CAD build for the part. Positions are in the model's coordinates, mm. A direction names the side the tool comes from. Give positions to 0.01 mm unless a question says otherwise; leave off trailing zeros. Order: outer loops, then holes, each group sorted by start corner. A loop starts at its lowest first (then second) coordinate and runs counter-clockwise, first axis right, second up.
Item 1: Band-saw the part on A-A on x = 48. Give the cut face in (y, z), plus the area to 3 significant figures.
Item 2: Band-saw the part on D-D on y = -14. Give the cut face in (x, z).
Item 3: Two-plate mould, pull along X, no slides. Class faces 6 (the flat face through (-3, 0, 6)), 7 (the cylindrical face through (-101.154, -39.08, -32.591)), 8 (the flat face through (-100.039, -47.546, 19.409)): released by +X, released by -X, zero draft, split by the parting line, or undercut.
Item 4: Band-saw the part on C-C on z = 3. Give the cut face in (x, y).
Item 5: Flat gauge pins, fed straight in: P1, Ø12, axis at y = -21, z = -22, coming from the +X side; P2, Ø10.5, axis at x = 25.5, z = 9.5, coming from the -Y side; P3, Ø8, axis at x = 1.5, y = -27.5, coming from the -Z side; P4, Ø5, axis at x = 21.5, y = -37, coming from the -Z side. Where does each tip first touch, or does it go through?
Item 6: Wall check: L1, parallel to Z at x = -92, y = -44; L2, parallel to Z at x = -74.5, y = -15; L3, parallel to Y at x = -19, z = 6. Give the ranges that are in metal, low to high.
Item 7: Which spindle directions (+Z, -Z, +X, -X, +Y, -Y) get a long thin tool onto all of the face, cutting with end or side? Do faces 1 (the flat face through (-95, -39, 15)), 2 (the flat face through (-78.604, -9.86, 19.409)), 3 (the flat face through (-93, -30, 13)), 4 (the flat face through (-78.604, -9.86, -19.227)), 5 (the flat face through (25, -22, 6)). Say none if no direction does.
Item 8: Band-saw the part on B-B on y = -47. Give the cut face in (x, z).
```python
from build123d import *

# Parameters (mm, degrees)
PAD_DEPTH    = 13
PAD001_DEPTH = 13
PAD002_DEPTH = 26
PAD003_DEPTH = 13
SKETCH004_R  = 6
POCKET_DEPTH = 54


with BuildPart() as part:
    # Sketch → Pad (new body)
    with BuildSketch(Plane.XY):
        Polygon((-84.297005, 0), (80.002995, 0), (80.002995, -20), (0, -20), (0, -22), (50, -22), (50, -33), (0, -33), (0, -35), (-5, -35), (-5, -20), (-72.75, -20), (-77.75, -28.660254), (-89.297005, -8.660254), align=None)
    extrude(amount=PAD_DEPTH)

    # Sketch001 (on Face16 of Pad) → Pad001 (join)
    with BuildSketch(Plane.XY.offset(13)):
        Polygon((-84.297005, 0), (-72.75, -20), (-91.5, -52.475953), (-108.820508, -42.475953), align=None)
    extrude(amount=PAD001_DEPTH)

    # Sketch002 (on Face4 of Pad001) → Pad002 (join)
    with BuildSketch(Plane(origin=(0, 0, 0), x_dir=(1, 0, 0), z_dir=(0, 0, -1))):
        Polygon((-77.75, 28.660254), (-89.297005, 8.660254), (-84.297005, 0), (-72.75, 20), align=None)
    extrude(amount=PAD002_DEPTH)

    # Sketch003 (on Face23 of Pad002) → Pad003 (join)
    with BuildSketch(Plane(origin=(0, 0, -26), x_dir=(1, 0, 0), z_dir=(0, 0, -1))):
        Polygon((-72.75, 20), (-91.5, 52.475953), (-108.820508, 42.475953), (-84.297005, 0), align=None)
    extrude(amount=PAD003_DEPTH)

    # Sketch004 (on Face31 of Pad003) → Pocket (cut)
    with BuildSketch(Plane(origin=(0, 0, -39), x_dir=(1, 0, 0), z_dir=(0, 0, -1))):
        with Locations((-95.160254, 38.815699)):
            Circle(SKETCH004_R)
    extrude(amount=-POCKET_DEPTH, mode=Mode.SUBTRACT)


solid = part.part
```
The answers:
1. outline: (-33, 0) - (-22, 0) - (-22, 13) - (-33, 13) - close; (-20, 0) - (0, 0) - (0, 13) - (-20, 13) - close
1. area: 403 mm2
2. outline: (-92.38, -39) - (-76.21, -39) - (-76.21, 0) - (80, 0) - (80, 13) - (-76.21, 13) - (-76.21, 26) - (-92.38, 26) - (-92.38, 13) - (-86.21, 13) - (-86.21, -26) - (-92.38, -26) - close
3. face 6: zero draft
3. face 7: undercut
3. face 8: released by -X
4. outline: (-89.3, -8.66) - (-77.75, -28.66) - (-72.75, -20) - (-5, -20) - (-5, -35) - (0, -35) - (0, -33) - (50, -33) - (50, -22) - (0, -22) - (0, -20) - (80, -20) - (80, 0) - (-84.3, 0) - close
5. P1: stops at x = -72.75
5. P2: stops at y = -33
5. P3: stops at z = 0
5. P4: passes through
6. L1: z = -39 to -26, 13 to 26
6. L2: z = 0 to 13
6. L3: y = -20 to 0
7. face 1: -Z
7. face 2: +Z, +X, +Y
7. face 3: -X, -Y
7. face 4: -Z, +X, +Y
7. face 5: +Z, -Z, +X
8. outline: (-100.98, -39) - (-88.34, -39) - (-88.34, -26) - (-100.98, -26) - close; (-100.98, 13) - (-88.34, 13) - (-88.34, 26) - (-100.98, 26) - close
